For this review, use the dimensioned drawing (mm, ordinates from the lowest corner) and the shaded views. A direction names the side the tool comes from. Round coordinates to 2 decimals unless told otherwise and drop trailing zeros. Write each loop counter-clockwise with the first axis right and the second up, starting at its lowest first coordinate (ties: lowest second). Pieces come first, ordered by that corner, then holes. Notation, with made-up numbers: M -30,30 L 7,30 A20 cw 7,43 Z; hole C 51,20 d1. An arc over 180 degrees is marked long. Use CSV: the item, a comma, the result in double quotes.
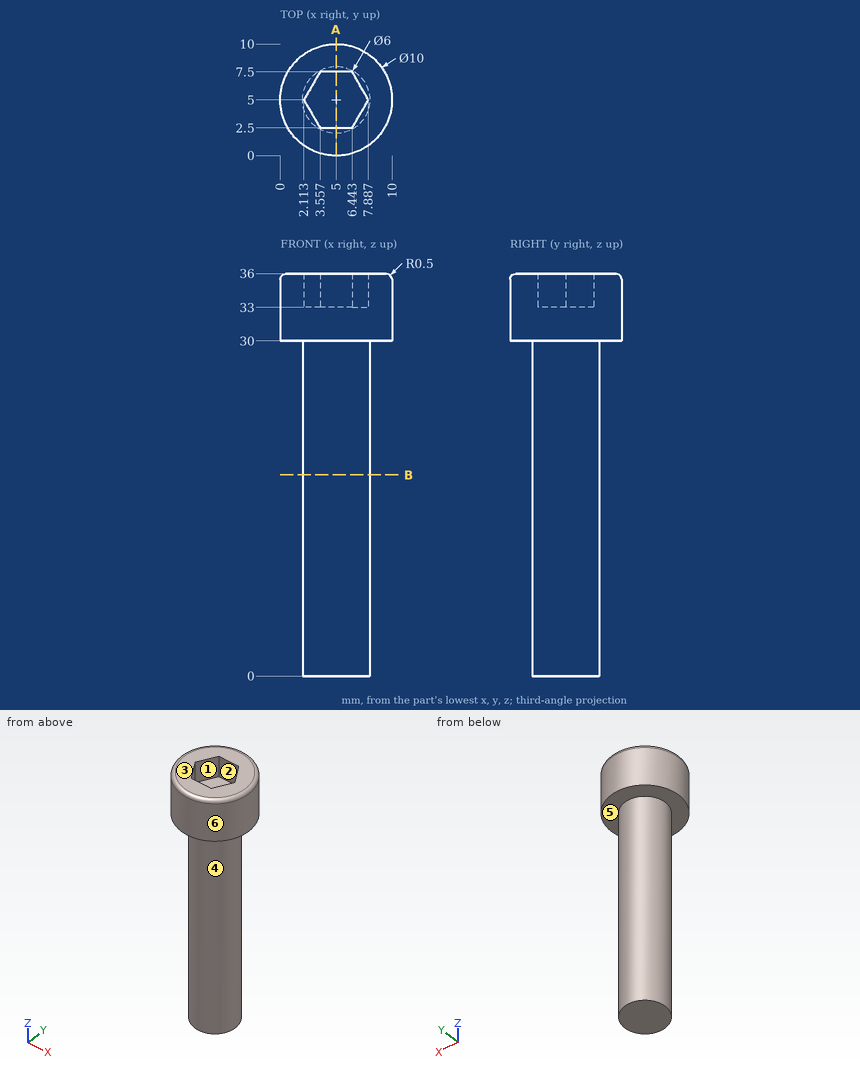
1) For pin 1 Ø5 at (x, y) = (6, 2.5) entering from -Z; pin 2 Ø1.5 at (x, z) = (3, 31) entering from +Y; pin 3 Ø3 at (y, z) = (8, 12) entering from -X; pin 4 Ø2.5 at (x, y) = (5, 4) entering from +Z, all flat-tipped, find the tip position at first contact; note any pin that passes through.
Answers:
pin 1,"z = 0"
pin 2,"y = 9.84"
pin 3,"x = 2.4"
pin 4,"z = 33"
2) Wall thickness on line 1 along Z through (x, y) = (6.25, 1.5); line 2 along Z through (x, y) = (3, 6); line 3 along X through (y, z) = (6, 7.5): over which ranges is each line inside the solid? List them lowest first. Write a range as [from, to].
Answers:
line 1,"[30, 36]"
line 2,"[0, 33]"
line 3,"[2.17, 7.83]"
3) Machinability: for the marked faces 5 and 6, which of the approach directions +Z, -Z, +X, -X, +Y, -Y give a long, thin tool a straight path to every point of the face, cutting with its end or side? Answer none if there is none.
Answers:
face 5,"-Z"
face 6,"+Z, -Z"
4) Add section B-B on z = 18. Write out the cut boundary in (x, y), then the cut area to 3 significant figures.
Answers:
outline,"C 5,5 d6"
area,"28.3 mm²"
5) Add section A-A on x = 5. Write out the cut boundary in (y, z).
Answers:
outline,"M 0,30 L 2,30 L 2,0 L 8,0 L 8,30 L 10,30 L 10,35.5 A0.5 ccw 9.5,36 L 7.5,36 L 7.5,33 L 2.5,33 L 2.5,36 L 0.5,36 A0.5 ccw 0,35.5 Z"
6) The part is to be moulded in two halves that separate along X. For the marked faces 1, 2, 3 and 4, say which applies: released by +X, released by -X, zero draft, split by the parting line, or undercut.
Answers:
face 1,"undercut"
face 2,"undercut"
face 3,"zero draft"
face 4,"split by the parting line"
